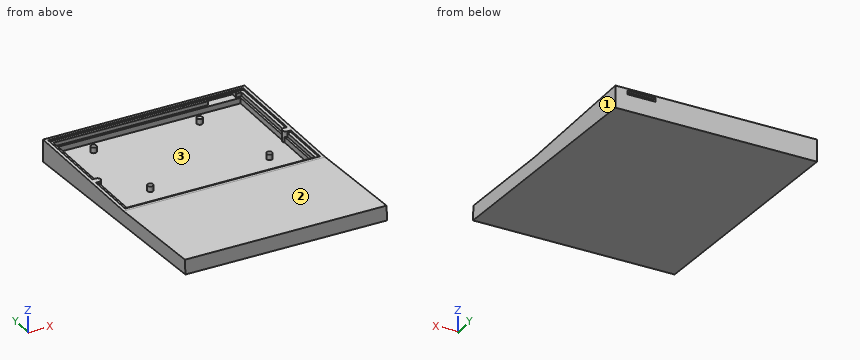
```python
from build123d import *

# Parameters (mm, degrees)
EXTRUDE_3_DEPTH     = 8.5
EXTRUDE_3_2_DEPTH   = 8.5
SKETCH_4_W          = 180.5019154
SKETCH_4_H          = 131.300307
EXTRUDE_5_DEPTH     = 10
EXTRUDE_6_DEPTH     = 5
SKETCH_8_W          = 25
SKETCH_8_H          = 6
CUT_EXTRUDE_1_DEPTH = 3.5
SKETCH_9_R          = 2.5
EXTRUDE_7_DEPTH     = 5
EXTRUDE_7_2_DEPTH   = 5
EXTRUDE_7_3_DEPTH   = 5
EXTRUDE_7_4_DEPTH   = 5
EXTRUDE_8_DEPTH     = 180.5019154


with BuildPart() as part:
    # Model → Extrude 3 (new body)
    with BuildSketch(Plane.XY):
        Polygon((565.397621393, -28.479593633), (562.397621393, -28.479593633), (562.397621393, -73.105300633), (393.895705993, -73.105300633), (393.895705993, -28.478893633), (390.895705993, -28.478893633), (390.895705993, -76.105300633), (565.397621393, -76.105300633), align=None)
    extrude(amount=EXTRUDE_3_DEPTH)



with BuildPart() as body_2:
    # Model → Extrude 3 2 (new body)
    with BuildSketch(Plane.XY):
        Polygon((393.895705993, -22.478893633), (393.895705993, 46.195006367), (562.397621393, 46.195006367), (562.397621393, -22.479593633), (565.397621393, -22.479593633), (565.397621393, 49.195006367), (390.895705993, 49.195006367), (390.895705993, -22.478893633), align=None)
    extrude(amount=EXTRUDE_3_2_DEPTH)


with BuildPart() as part_1:
    add(part.part)

    add(body_2.part)  # Extrude 5 merges body 2
    # Sketch 4 → Extrude 5 (add)
    with BuildSketch(Plane(origin=(0, 0, 0), x_dir=(-1, 0, 0), z_dir=(0, 0, -1))):
        with Locations((-478.146663693, -13.455147133)):
            Rectangle(SKETCH_4_W, SKETCH_4_H)
        with BuildLine():
            ThreePointArc((-562.397621393, -28.479593633), (-559.397621393, -25.479593633), (-562.397621393, -22.479593633))
            Line((-562.397621393, -22.479593633), (-565.397621393, -22.479593633))
            Line((-565.397621393, -22.479593633), (-565.397621393, 49.195006367))
            Line((-565.397621393, 49.195006367), (-390.895705993, 49.195006367))
            Line((-390.895705993, 49.195006367), (-390.895705993, -22.478893633))
            Line((-390.895705993, -22.478893633), (-393.895705993, -22.478893633))
            ThreePointArc((-393.895705993, -22.478893633), (-396.895705993, -25.478893633), (-393.895705993, -28.478893633))
            Line((-393.895705993, -28.478893633), (-390.895705993, -28.478893633))
            Line((-390.895705993, -28.478893633), (-390.895705993, -76.105300633))
            Line((-390.895705993, -76.105300633), (-565.397621393, -76.105300633))
            Line((-565.397621393, -76.105300633), (-565.397621393, -28.479593633))
            Line((-565.397621393, -28.479593633), (-562.397621393, -28.479593633))
        make_face(mode=Mode.SUBTRACT)
    extrude(amount=-EXTRUDE_5_DEPTH)

    # Sketch 5 → Extrude 6 (add)
    with BuildSketch(Plane(origin=(0, 0, 0), x_dir=(-1, 0, 0), z_dir=(0, 0, -1))):
        with BuildLine():
            Line((-562.397621393, 46.195006367), (-562.397621393, -22.479593633))
            ThreePointArc((-562.397621393, -22.479593633), (-561.327155124, -22.677076556), (-560.397621393, -23.243525656))
            Line((-560.397621393, -23.243525656), (-560.397621393, 44.195006367))
            Line((-560.397621393, 44.195006367), (-395.895705993, 44.195006367))
            Line((-395.895705993, 44.195006367), (-395.895705993, -23.242825656))
            ThreePointArc((-395.895705993, -23.242825656), (-394.966172262, -22.676376556), (-393.895705993, -22.478893633))
            Line((-393.895705993, -22.478893633), (-393.895705993, 46.195006367))
            Line((-393.895705993, 46.195006367), (-562.397621393, 46.195006367))
        make_face()
        with BuildLine():
            Line((-560.397621393, -71.105300633), (-560.397621393, -27.715661611))
            ThreePointArc((-560.397621393, -27.715661611), (-561.327155124, -28.28211071), (-562.397621393, -28.479593633))
            Line((-562.397621393, -28.479593633), (-562.397621393, -73.105300633))
            Line((-562.397621393, -73.105300633), (-393.895705993, -73.105300633))
            Line((-393.895705993, -73.105300633), (-393.895705993, -28.478893633))
            ThreePointArc((-393.895705993, -28.478893633), (-394.966172262, -28.28141071), (-395.895705993, -27.714961611))
            Line((-395.895705993, -27.714961611), (-395.895705993, -71.105300633))
            Line((-395.895705993, -71.105300633), (-560.397621393, -71.105300633))
        make_face()
    extrude(amount=-EXTRUDE_6_DEPTH)

    # Sketch 8 → Cut-Extrude 1 (cut)
    with BuildSketch(Plane.XY.offset(5)):
        with Locations((544.897621393, 49.195006367)):
            Rectangle(SKETCH_8_W, SKETCH_8_H)
    extrude(amount=CUT_EXTRUDE_1_DEPTH, mode=Mode.SUBTRACT)



with BuildPart() as body_2_2:
    # Sketch 9 → Extrude 7 (new body)
    with BuildSketch(Plane(origin=(0, 0, 0), x_dir=(-1, 0, 0), z_dir=(0, 0, -1))):
        with Locations((-430.805705993, -44.525300633)):
            Circle(SKETCH_9_R)
    extrude(amount=-EXTRUDE_7_DEPTH)


with BuildPart() as body_3:
    # Sketch 9 → Extrude 7 2 (new body)
    with BuildSketch(Plane(origin=(0, 0, 0), x_dir=(-1, 0, 0), z_dir=(0, 0, -1))):
        with Locations((-537.477621393, -44.525300633)):
            Circle(SKETCH_9_R)
    extrude(amount=-EXTRUDE_7_2_DEPTH)


with BuildPart() as body_4:
    # Sketch 9 → Extrude 7 3 (new body)
    with BuildSketch(Plane(origin=(0, 0, 0), x_dir=(-1, 0, 0), z_dir=(0, 0, -1))):
        with Locations((-421.895705993, 31.665006367)):
            Circle(SKETCH_9_R)
    extrude(amount=-EXTRUDE_7_3_DEPTH)


with BuildPart() as body_5:
    # Sketch 9 → Extrude 7 4 (new body)
    with BuildSketch(Plane(origin=(0, 0, 0), x_dir=(-1, 0, 0), z_dir=(0, 0, -1))):
        with Locations((-516.895705993, 31.665006367)):
            Circle(SKETCH_9_R)
    extrude(amount=-EXTRUDE_7_4_DEPTH)


with BuildPart() as part_2:
    add(part_1.part)

    add(body_2_2.part)  # Extrude 8 merges body 2 2

    add(body_3.part)  # Extrude 8 merges body 3

    add(body_4.part)  # Extrude 8 merges body 4

    add(body_5.part)  # Extrude 8 merges body 5
    # Sketch 10 → Extrude 8 (add)
    with BuildSketch(Plane.ZY.offset(-387.895705993)):
        Polygon((2.251411672, -179.64862154), (-9.898998007, 52.195006367), (0, 52.195006367), (0, -79.105300633), (10, -79.105300633), (15.233595624, -178.968254109), align=None)
    extrude(amount=-EXTRUDE_8_DEPTH)


solid = part_2.part
```
Part model, mm, in its own coordinate system. Face numbers are marked on the shaded views. Round coordinates to 2 decimals unless told otherwise and drop trailing zeros. Loops run counter-clockwise (first coordinate to the right, second up) from the corner with the lowest first, then second, coordinate; pieces in that order, holes last. Notation, with made-up numbers: (-38, 64) -> (-9, 64) arc R27 ccw to (-9, 98) -> close; hole circle Ø9 at (60, -34.5). An arc over 180 degrees is marked (long way). Use one line per item in the form item = value. Start each with the question number.
Item 1: Drill centre lines: line 1 along X through (y, z) = (-7, 9.5); line 2 along Y through (x, z) = (418, 5.5) (3 decimals); line 3 along Z through (x, y) = (470.5, -100.5). Where is each one in solid material? Low to high.
Item 2: Band-saw the part on B-B (x = 452.5). List the corners of the cut face in (y, z) (3 decimals), plus the area to 3 significant figures.
Item 3: Drop flat-ended pins along their axis: pin 1 Ø2 at (y, z) = (-25, 11.5) entering from +X; pin 2 Ø2.5 at (x, y) = (562.5, 8) entering from +Z; pin 3 Ø1.6 at (x, z) = (563.5, 9.5) entering from -Y; pin 4 Ø22.5 at (x, y) = (457, -50) entering from +Z. Give the stop position or say it passes through.
Item 4: Band-saw the part on D-D (y = 19). List the corners of the cut face in (x, z).
Item 5: Band-saw the part on C-C (y = -17). List the corners of the cut face in (x, z), plus the area to 3 significant figures.
Item 6: Band-saw the part on A-A (x = 545). List the corners of the cut face in (y, z) (3 decimals).
Item 7: Two-plate mould, pull along X, no slides. Class the marked faces 1, 2 and 3: released by +X, released by -X, zero draft, split by the parting line, or undercut.
Data:
q1.line_1 = 387.9 to 390.9, 565.4 to 568.4
q1.line_2 = -179.478 to -73.105, 46.195 to 52.195
q1.line_3 = -1.9 to 11.12
q2.outline = (-179.649, 2.251) -> (52.195, -9.899) -> (52.195, 10) -> (49.195, 10) -> (49.195, 8.5) -> (46.195, 8.5) -> (46.195, 5) -> (44.195, 5) -> (44.195, 0) -> (-71.105, 0) -> (-71.105, 5) -> (-73.105, 5) -> (-73.105, 8.5) -> (-76.105, 8.5) -> (-76.105, 10) -> (-79.105, 10) -> (-178.968, 15.234) -> close
q2.area = 2,280 mm^2
q3.pin_1 = through
q3.pin_2 = 8.5
q3.pin_3 = -179.31
q3.pin_4 = 0
q4.outline = (387.9, -8.16) -> (568.4, -8.16) -> (568.4, 10) -> (565.4, 10) -> (565.4, 8.5) -> (562.4, 8.5) -> (562.4, 5) -> (560.4, 5) -> (560.4, 0) -> (395.9, 0) -> (395.9, 5) -> (393.9, 5) -> (393.9, 8.5) -> (390.9, 8.5) -> (390.9, 10) -> (387.9, 10) -> close
q5.outline = (387.9, -6.27) -> (568.4, -6.27) -> (568.4, 10) -> (565.4, 10) -> (565.4, 8.5) -> (562.4, 8.5) -> (562.4, 5) -> (560.4, 5) -> (560.4, 0) -> (395.9, 0) -> (395.9, 5) -> (393.9, 5) -> (393.9, 8.5) -> (390.9, 8.5) -> (390.9, 10) -> (387.9, 10) -> close
q5.area = 1,260 mm^2
q6.outline = (-179.649, 2.251) -> (52.195, -9.899) -> (52.195, 5) -> (44.195, 5) -> (44.195, 0) -> (-71.105, 0) -> (-71.105, 5) -> (-73.105, 5) -> (-73.105, 8.5) -> (-76.105, 8.5) -> (-76.105, 10) -> (-79.105, 10) -> (-178.968, 15.234) -> close; (49.195, 8.5) -> (52.195, 8.5) -> (52.195, 10) -> (49.195, 10) -> close
q7.face_1 = released by +X
q7.face_2 = zero draft
q7.face_3 = undercut
